from build123d import *

# Parameters (mm, degrees)
SKETCH1_R           = 25.4
SKETCH1_R_2         = 2.5527
BOSS_EXTRUDE1_DEPTH = 3.175


with BuildPart() as part:
    # Sketch1 → Boss-Extrude1 (new body)
    with BuildSketch(Plane(origin=(0, 0, 0), x_dir=(1, 0, 0), z_dir=(0, 1, 0))):
        with BuildLine():
            Line((0, 0), (-381, 0))
            Line((-381, 0), (-381, -289.5092))
            ThreePointArc((-381, -289.5092), (-380.883021338, -292.492501864), (-380.532803674, -295.457484428))
            Line((-380.532803674, -295.457484428), (-374.89739058, -331.110855945))
            ThreePointArc((-374.89739058, -331.110855945), (-371.869518463, -336.696056706), (-366.003133246, -339.134909219))
            Line((-366.003133246, -339.134909219), (-341.613815414, -340.452811597))
            ThreePointArc((-341.613815414, -340.452811597), (-290.115080631, -324.037048347), (-262.459915955, -277.595807687))
            Line((-262.459915955, -277.595807687), (-228.02117539, -82.284004431))
            ThreePointArc((-228.02117539, -82.284004431), (-190.5, -50.8), (-152.97882461, -82.284004431))
            Line((-152.97882461, -82.284004431), (-118.540084045, -277.595807687))
            ThreePointArc((-118.540084045, -277.595807687), (-90.884919369, -324.037048347), (-39.386184586, -340.452811597))
            Line((-39.386184586, -340.452811597), (-14.996866754, -339.134909219))
            ThreePointArc((-14.996866754, -339.134909219), (-9.130481537, -336.696056706), (-6.10260942, -331.110855945))
            Line((-6.10260942, -331.110855945), (-0.467196326, -295.457484428))
            ThreePointArc((-0.467196326, -295.457484428), (-0.116978662, -292.492501864), (0, -289.5092))
            Line((0, -289.5092), (0, 0))
        make_face()
        with Locations(Location((-342.9, -190.5, 0), (0, 0, 270))):
            Circle(SKETCH1_R, mode=Mode.SUBTRACT)
        with Locations(Location((-350.506535266, -149.065461092, 0), (0, 0, 270))):
            Circle(SKETCH1_R_2, mode=Mode.SUBTRACT)
        with Locations(Location((-342.9, -289.5092, 0), (0, 0, 270))):
            Circle(SKETCH1_R, mode=Mode.SUBTRACT)
        with Locations(Location((-365.489189661, -329.623784838, 0), (0, 0, 270))):
            Circle(SKETCH1_R_2, mode=Mode.SUBTRACT)
        with Locations(Location((-366.035610617, -233.842290605, 0), (0, 0, 270))):
            Circle(SKETCH1_R_2, mode=Mode.SUBTRACT)
        with Locations(Location((-315.890976945, -241.97590689, 0), (0, 0, 270))):
            Circle(SKETCH1_R_2, mode=Mode.SUBTRACT)
        with Locations(Location((-65.109023055, -241.97590689, 0), (0, 0, 90))):
            Circle(SKETCH1_R_2, mode=Mode.SUBTRACT)
        with Locations(Location((-14.964389383, -233.842290605, 0), (0, 0, 90))):
            Circle(SKETCH1_R_2, mode=Mode.SUBTRACT)
        with Locations(Location((-15.510810339, -329.623784838, 0), (0, 0, 90))):
            Circle(SKETCH1_R_2, mode=Mode.SUBTRACT)
        with Locations(Location((-38.1, -289.5092, 0), (0, 0, 90))):
            Circle(SKETCH1_R, mode=Mode.SUBTRACT)
        with Locations(Location((-30.493464734, -149.065461092, 0), (0, 0, 90))):
            Circle(SKETCH1_R_2, mode=Mode.SUBTRACT)
        with Locations(Location((-38.1, -190.5, 0), (0, 0, 90))):
            Circle(SKETCH1_R, mode=Mode.SUBTRACT)
    extrude(amount=BOSS_EXTRUDE1_DEPTH)


solid = part.part
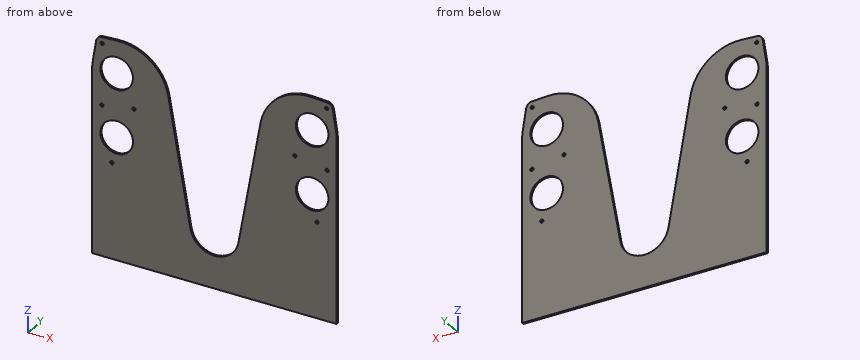
Can you work these out from the model? Positions are in its coordinate system, mm. Coordinates: 2 decimals unless noted, no trailing zeros. Order: outer loops, then holes, each group sorted by start corner. A loop starts at its lowest first (then second) coordinate and runs counter-clockwise, first axis right, second up. Notation, with made-up numbers: (-22.75, 32.5) - (13.25, 32.5) arc R32 cw to (13.25, 69.5) - close; hole circle Ø7 at (29, 86.25). An arc over 180 degrees is marked (long way). Answer as a JSON object with one key per item and string values. Group by question number.
Q1. Imagine slicing it at C-C (z = 161). Please give me the cut outline in (x, y) (3 decimals).
Q2. Imagine slicing it at B-B (y = 0.85). Give the number of separate pieces and of enclosed holes in the cut face, and give its area (3 significant figures).
Q3. Imagine slicing it at D-D (x = -198). Please give me the cut outline in (y, z) (3 decimals), and give its area (3 significant figures).
Q4. Imagine slicing it at A-A (z = 269). Please give me the cut outline in (x, y) (3 decimals), and give its area (3 significant figures).
Q5. I need wall thicknesses on line 1 (X direction, y = 2.85, z = 176.5); line 2 (Z direction, x = -352, y = 2); line 3 (X direction, y = 2.85, z = 209.5). Which ranges of each line are inside material? Lowest first, please. Write a range as from..to.
Q6. Will this pin go through, and if not, where does the flat tip stop? P1, Ø6, axis at x = -99, z = 183, coming from the -Y side.
Determined:
{
 "1": {"outline": "(-381, 0) - (-241.901, 0) - (-241.901, 3.175) - (-381, 3.175) - close; (-139.099, 0) - (0, 0) - (0, 3.175) - (-139.099, 3.175) - close"},
 "2": {"separate pieces": "1", "enclosed holes": "12", "area": "86,500 mm2"},
 "3": {"outline": "(0, 0) - (3.175, 0) - (3.175, 51.545) - (0, 51.545) - close", "area": "164 mm2"},
 "4": {"outline": "(-381, 0) - (-357.884, 0) - (-357.884, 3.175) - (-381, 3.175) - close; (-327.916, 0) - (-260.944, 0) - (-260.944, 3.175) - (-327.916, 3.175) - close; (-120.056, 0) - (-53.084, 0) - (-53.084, 3.175) - (-120.056, 3.175) - close; (-23.116, 0) - (0, 0) - (0, 3.175) - (-23.116, 3.175) - close", "area": "572 mm2"},
 "5": {"line 1": "x = -381..-364.09, -321.71..-244.63, -136.37..-59.29, -16.91..0", "line 2": "z = 0..147, 151.14..166.79, 214.21..265.8, 313.22..339.89", "line 3": "x = -381..-359.76, -326.04..-250.45, -130.55..-54.96, -21.24..0"},
 "6": {"P1": "stops at y = 0"}
}
